```python
from build123d import *

# Parameters (mm, degrees)
SKETCH2_R           = 4.25
SKETCH2_R_2         = 2.75
BOSS_EXTRUDE1_DEPTH = 6.5
SKETCH3_W           = 20
SKETCH3_H           = 30
BOSS_EXTRUDE2_DEPTH = 6.5
SKETCH4_R           = 2.75
CUT_EXTRUDE1_DEPTH  = 289.885357884
SKETCH5_W           = 0.4
SKETCH5_H           = 30
BOSS_EXTRUDE3_DEPTH = 6.5
SKETCH6_R           = 2.75
SKETCH6_R_2         = 4
BOSS_EXTRUDE4_DEPTH = 6.5
SKETCH9_W           = 23
SKETCH9_H           = 30
BOSS_EXTRUDE6_DEPTH = 5
BOSS_EXTRUDE7_DEPTH = 14
FILLET1_START       = -17
FILLET1_DEPTH       = 24
FILLET1_START_2     = -16.5
FILLET1_2_DEPTH     = 6.5
FILLET1_3_DEPTH     = 6.5


with BuildPart() as part:
    # Sketch2 → Boss-Extrude1 (new body)
    with BuildSketch(Plane.XY):
        with BuildLine():
            ThreePointArc((12.5, 235.505102572), (0, 287.5), (-12.5, 235.505102572))
            Line((-12.5, 235.505102572), (-12.5, 190))
            ThreePointArc((-12.5, 190), (0, 177.5), (12.5, 190))
            Line((12.5, 190), (12.5, 235.505102572))
        make_face()
        with Locations(Location((0, 260, 0), (0, 0, 180))):
            Circle(SKETCH2_R, mode=Mode.SUBTRACT)
        with Locations(Location((0, 225, 0), (0, 0, 180))):
            Circle(SKETCH2_R_2, mode=Mode.SUBTRACT)
        with Locations(Location((0, 190, 0), (0, 0, 180))):
            Circle(SKETCH2_R_2, mode=Mode.SUBTRACT)
    extrude(amount=BOSS_EXTRUDE1_DEPTH)

    # Sketch3 → Boss-Extrude2 (add)
    with BuildSketch(Plane.XY.offset(6.5)):
        with Locations((-10, 210)):
            Rectangle(SKETCH3_W, SKETCH3_H)
    extrude(amount=-BOSS_EXTRUDE2_DEPTH)

    # Sketch4 → Cut-Extrude1 (cut, through all)
    with BuildSketch(Plane.XY.offset(6.5)):
        with Locations(Location((0, 225, 0), (0, 0, 180))):
            Circle(SKETCH4_R)
    extrude(amount=-CUT_EXTRUDE1_DEPTH, mode=Mode.SUBTRACT)

    # Sketch5 → Boss-Extrude3 (add)
    with BuildSketch(Plane.XY.offset(6.5)):
        with Locations((-20.2, 210)):
            Rectangle(SKETCH5_W, SKETCH5_H)
    extrude(amount=-BOSS_EXTRUDE3_DEPTH)



with BuildPart() as body_2:
    # Sketch6 → Boss-Extrude4 (new body)
    with BuildSketch(Plane(origin=(0, 0, -10), x_dir=(-1, 0, 0), z_dir=(0, 0, -1))):
        with BuildLine():
            Line((12.5, 190), (12.5, 195))
            Line((12.5, 195), (20.4, 195))
            Line((20.4, 195), (20.4, 225))
            Line((20.4, 225), (12.5, 225))
            Line((12.5, 225), (12.5, 235.505102572))
            ThreePointArc((12.5, 235.505102572), (0, 287.5), (-12.5, 235.505102572))
            Line((-12.5, 235.505102572), (-12.5, 190))
            ThreePointArc((-12.5, 190), (0, 177.5), (12.5, 190))
        make_face()
        with Locations((0, 190)):
            Circle(SKETCH6_R, mode=Mode.SUBTRACT)
        with Locations((0, 225)):
            Circle(SKETCH6_R, mode=Mode.SUBTRACT)
        with Locations(Location((0, 260, 0), (0, 0, 180))):
            Circle(SKETCH6_R_2, mode=Mode.SUBTRACT)
    extrude(amount=BOSS_EXTRUDE4_DEPTH)


with BuildPart() as part_1:
    add(part.part)

    add(body_2.part)  # Boss-Extrude6 merges body 2
    # Sketch9 → Boss-Extrude6 (add)
    with BuildSketch(Plane.ZY.offset(20.4)):
        with Locations((-5, 210)):
            Rectangle(SKETCH9_W, SKETCH9_H)
    extrude(amount=BOSS_EXTRUDE6_DEPTH)

    # Sketch10 → Boss-Extrude7 (add)
    with BuildSketch(Plane(origin=(0, 0, 0), x_dir=(-1, 0, 0), z_dir=(0, 0, -1))):
        with BuildLine():
            ThreePointArc((20.4, 241.558470779), (25.406687144, 249.47620561), (27.465108704, 258.615152031))
            Line((27.465108704, 258.615152031), (23.211774901, 254.361818228))
            ThreePointArc((23.211774901, 254.361818228), (21.130756488, 251.24735408), (20.4, 247.573593129))
            Line((20.4, 247.573593129), (20.4, 241.558470779))
        make_face()
    extrude(amount=BOSS_EXTRUDE7_DEPTH)

    # Fillet1: read off the stored shape, not the designer's step
    # Fillet1 outline → Fillet1 (cut)
    with BuildSketch(Plane.XY.offset(FILLET1_START)):
        with BuildLine():
            ThreePointArc((-20.4, 195), (-23.935533906, 196.464466094), (-25.4, 200))
            Line((-25.4, 200), (-25.4, 195))
            Line((-25.4, 195), (-20.4, 195))
        make_face()
        with BuildLine():
            ThreePointArc((-25.4, 220), (-23.935533906, 223.535533906), (-20.4, 225))
            Line((-20.4, 225), (-25.4, 225))
            Line((-25.4, 225), (-25.4, 220))
        make_face()
    extrude(amount=FILLET1_DEPTH, mode=Mode.SUBTRACT)

    # Fillet1 2 outline → Fillet1 2 (add)
    with BuildSketch(Plane.XY.offset(FILLET1_START_2)):
        with BuildLine():
            Line((12.5, 235.505102572), (12.5, 232.613872125))
            ThreePointArc((12.5, 232.613872125), (13.114709903, 235.015794432), (14.807692308, 236.827122567))
            ThreePointArc((14.807692308, 236.827122567), (13.669837198, 236.138198916), (12.5, 235.505102572))
        make_face()
        with BuildLine():
            Line((-12.5, 195), (-17.5, 195))
            ThreePointArc((-17.5, 195), (-13.964466094, 193.535533906), (-12.5, 190))
            Line((-12.5, 190), (-12.5, 195))
        make_face()
        with BuildLine():
            Line((-12.5, 225), (-12.5, 230))
            ThreePointArc((-12.5, 230), (-13.964466094, 226.464466094), (-17.5, 225))
            Line((-17.5, 225), (-12.5, 225))
        make_face()
        with BuildLine():
            ThreePointArc((-12.5, 235.505102572), (-13.669837198, 236.138198916), (-14.807692308, 236.827122567))
            ThreePointArc((-14.807692308, 236.827122567), (-13.114709903, 235.015794432), (-12.5, 232.613872125))
            Line((-12.5, 232.613872125), (-12.5, 235.505102572))
        make_face()
    extrude(amount=FILLET1_2_DEPTH)

    # Fillet1 3 outline → Fillet1 3 (add)
    with BuildSketch(Plane.XY):
        with BuildLine():
            Line((12.5, 235.505102572), (12.5, 232.613872125))
            ThreePointArc((12.5, 232.613872125), (13.114709903, 235.015794432), (14.807692308, 236.827122567))
            ThreePointArc((14.807692308, 236.827122567), (13.669837198, 236.138198916), (12.5, 235.505102572))
        make_face()
        with BuildLine():
            Line((-12.5, 195), (-17.5, 195))
            ThreePointArc((-17.5, 195), (-13.964466094, 193.535533906), (-12.5, 190))
            Line((-12.5, 190), (-12.5, 195))
        make_face()
        with BuildLine():
            Line((-12.5, 225), (-12.5, 230))
            ThreePointArc((-12.5, 230), (-13.964466094, 226.464466094), (-17.5, 225))
            Line((-17.5, 225), (-12.5, 225))
        make_face()
        with BuildLine():
            ThreePointArc((-12.5, 235.505102572), (-13.669837198, 236.138198916), (-14.807692308, 236.827122567))
            ThreePointArc((-14.807692308, 236.827122567), (-13.114709903, 235.015794432), (-12.5, 232.613872125))
            Line((-12.5, 232.613872125), (-12.5, 235.505102572))
        make_face()
    extrude(amount=FILLET1_3_DEPTH)


solid = part_1.part
```
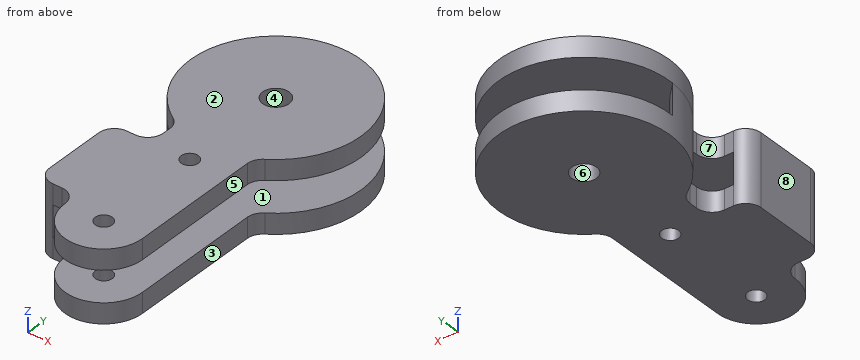
CAD build for the part. Positions are in the model's coordinates, mm. Face numbers are marked on the shaded views. A direction names the side the tool comes from. Give positions to 0.01 mm unless a question says otherwise; leave off trailing zeros. Order: outer loops, then holes, each group sorted by start corner. A loop starts at its lowest first (then second) coordinate and runs counter-clockwise, first axis right, second up.
(1) Flat gauge pins, fed straight in: pin 1 (1.5 mm diameter, centred on x = 16.5, z = -0.5, fed in from +Y); pin 2 (10 mm diameter, centred on y = 201.5, z = 0, fed in from +X); pin 3 (10 mm diameter, centred on y = 210, z = -2, fed in from -X). Where does each tip first touch, or does it go through?
(2) Saw through at C-C, the plane x = 0. State how many separate pieces and enclosed holes the cut face has, then the cut area to 3 significant figures.
(3) Saw through at B-B, the plane y = 260. Give the cut face in (x, z), then the cut area to 3 significant figures.
(4) Saw through at A-A, the plane z = -4.25. Give the cut face in (x, y).
(5) Mould opens along Z. For the marked faces 1, 2 and 3 say: released by +Z, released by -Z, zero draft, split by the parting line, or undercut.
(6) Drill centre lines: L1, parallel to Y at x = 0, z = -13.75; L2, parallel to Y at x = 0, z = 2.5; L3, parallel to Z at x = 19, y = 260. Where is each one in solid material? Low to high.
(7) Tool access for the marked faces 4, 5, 6, 7 and 8: list every direction of +Z, -Z, +X, -X, +Y, -Y with a clear straight run to the whole face (end or side of a thin tool).
(8) Saw through at D-D, the plane y = 271. Give the cut face in (x, z).
Results found:
1. pin 1: stops at y = 282.41
1. pin 2: stops at x = 12.5
1. pin 3: stops at x = -25.4
2. separate pieces: 8
2. enclosed holes: 0
2. area: 1,180 mm2
3. outline: (-27.5, -16.5) - (-4, -16.5) - (-4, -10) - (-27.5, -10) - close; (-27.5, 0) - (-4.25, 0) - (-4.25, 6.5) - (-27.5, 6.5) - close; (4, -16.5) - (27.5, -16.5) - (27.5, -10) - (4, -10) - close; (4.25, 0) - (27.5, 0) - (27.5, 6.5) - (4.25, 6.5) - close
3. area: 608 mm2
4. outline: (-27.47, 258.62) arc R27.5 ccw to (-20.4, 241.56) - (-20.4, 247.57) arc R9.6 ccw to (-23.21, 254.36) - close; (-25.4, 200) arc R5 ccw to (-20.4, 195) - (-20.4, 225) arc R5 ccw to (-25.4, 220) - close
5. face 1: undercut
5. face 2: released by +Z
5. face 3: zero draft
6. L1: y = 177.5 to 187.25, 192.75 to 222.25, 227.75 to 256, 264 to 287.5
6. L2: y = 177.5 to 187.25, 192.75 to 222.25, 227.75 to 255.75, 264.25 to 287.5
6. L3: z = -16.5 to -10, 0 to 6.5
7. face 4: +Z
7. face 5: +Z, -Z, +X, -Y
7. face 6: +Z, -Z
7. face 7: +Z, -Z, -X
7. face 8: +Z, -Z, -X, -Y
8. outline: (-25.2, -16.5) - (25.2, -16.5) - (25.2, -10) - (-25.2, -10) - close; (-25.2, 0) - (25.2, 0) - (25.2, 6.5) - (-25.2, 6.5) - close
